The model under review builds one solid part; all positions refer to its coordinate system, in mm. A direction names the side the tool comes from. Round coordinates to 2 decimals unless told otherwise and drop trailing zeros. Order: outer loops, then holes, each group sorted by start corner. A loop starts at its lowest first (then second) coordinate and runs counter-clockwise, first axis right, second up.
from build123d import *

# Parameters (mm, degrees)
ROTATION1_ANGLE                                      = 180
FORMSENKUNG_F_R_M3_SENKSCHRAUBE_MIT_INNE_D           = 1.6
FORMSENKUNG_F_R_M3_SENKSCHRAUBE_MIT_INNE_DEPTH       = 12
FORMSENKUNG_F_R_M3_SENKSCHRAUBE_MIT_INNE_CSINK_D     = 3.9
FORMSENKUNG_F_R_M3_SENKSCHRAUBE_MIT_INNE_CSINK_ANGLE = 90
FORMSENKUNG_F_R_M3_SENKSCHRAUBE_MIT_INNE_TIP         = 0.480688495
SKIZZE12_R                                           = 1
SCHNITT_LINEAR_AUSTRAGEN1_DEPTH                      = 10.5
SKIZZE9_R                                            = 3
SCHNITT_LINEAR_AUSTRAGEN2_DEPTH                      = 19
SKIZZE9_5_R                                          = 3.5
SCHNITT_LINEAR_AUSTRAGEN3_DEPTH                      = 16.5
SCHNITT_LINEAR_AUSTRAGEN5_DEPTH                      = 4
STIRNSENKUNG_F_R_M3_D_NNKOPF_ZYLINDERSCH_D           = 3.2
STIRNSENKUNG_F_R_M3_D_NNKOPF_ZYLINDERSCH_CBORE_D     = 5.6
STIRNSENKUNG_F_R_M3_D_NNKOPF_ZYLINDERSCH_CBORE_DEPTH = 2.1


with BuildPart() as part:
    # Skizze4 → Rotation1 (revolve, symmetric)
    with BuildSketch(Plane.XY) as rotation1_sk:
        Polygon((3.5, 20), (-4, 20), (-4, 13), (5.5, 13), (5.5, 22), (3.5, 22), align=None)
    revolve(axis=Axis((0, 0, 0), (-1, 0, 0)), revolution_arc=ROTATION1_ANGLE / 2)
    revolve(rotation1_sk.sketch, axis=Axis((0, 0, 0), (1, 0, 0)), revolution_arc=ROTATION1_ANGLE / 2)

    # Formsenkung f_r M3 Senkschraube mit Inne
    with Locations(Plane(origin=(5.5, 0, 0), x_dir=(0, 0, -1), z_dir=(1, 0, 0))):
        with Locations((6.696960066, 16.167891819), (-16.167891819, 6.696960066), (-6.696960066, 16.167891819), (16.167891819, 6.696960066)):
            CounterSinkHole(FORMSENKUNG_F_R_M3_SENKSCHRAUBE_MIT_INNE_D / 2, FORMSENKUNG_F_R_M3_SENKSCHRAUBE_MIT_INNE_CSINK_D / 2, depth=FORMSENKUNG_F_R_M3_SENKSCHRAUBE_MIT_INNE_DEPTH, counter_sink_angle=FORMSENKUNG_F_R_M3_SENKSCHRAUBE_MIT_INNE_CSINK_ANGLE)
            with Locations((0, 0, -(FORMSENKUNG_F_R_M3_SENKSCHRAUBE_MIT_INNE_DEPTH + FORMSENKUNG_F_R_M3_SENKSCHRAUBE_MIT_INNE_TIP / 2))):  # 118° drill point
                Cone(0, FORMSENKUNG_F_R_M3_SENKSCHRAUBE_MIT_INNE_D / 2, FORMSENKUNG_F_R_M3_SENKSCHRAUBE_MIT_INNE_TIP, mode=Mode.SUBTRACT)

    # Skizze12 → Schnitt-Linear austragen1 (cut, through all)
    with BuildSketch(Plane(origin=(5.5, 0, 0), x_dir=(0, 0, -1), z_dir=(1, 0, 0))):
        with Locations((-6.696960066, 16.167891819)):
            Circle(SKIZZE12_R)
        with Locations((6.696960066, 16.167891819)):
            Circle(SKIZZE12_R)
        with Locations((16.167891819, 6.696960066)):
            Circle(SKIZZE12_R)
        with Locations((-16.167891819, 6.696960066)):
            Circle(SKIZZE12_R)
    extrude(amount=-SCHNITT_LINEAR_AUSTRAGEN1_DEPTH, mode=Mode.SUBTRACT)

    # Skizze9 → Schnitt-Linear austragen2 (cut, symmetric)
    with BuildSketch(Plane(origin=(0, 0, 0), x_dir=(1, 0, 0), z_dir=(0, 1, 0))):
        Circle(SKIZZE9_R)
    extrude(amount=SCHNITT_LINEAR_AUSTRAGEN2_DEPTH, both=True, mode=Mode.SUBTRACT)

    # Skizze9_5 → Schnitt-Linear austragen3 (cut, symmetric)
    with BuildSketch(Plane(origin=(0, 0, 0), x_dir=(1, 0, 0), z_dir=(0, 1, 0))):
        Circle(SKIZZE9_5_R)
    extrude(amount=SCHNITT_LINEAR_AUSTRAGEN3_DEPTH, both=True, mode=Mode.SUBTRACT)

    # Skizze15 → Schnitt-Linear austragen5 (cut)
    with BuildSketch(Plane(origin=(5.5, 0, 0), x_dir=(0, 0, -1), z_dir=(1, 0, 0))):
        Polygon((-14.883419246, 2.8), (-18.116580754, 2.8), (-19.733161507, 0), (-18.116580754, -2.8), (-14.883419246, -2.8), (-13.266838493, 0), align=None)
        Polygon((13.266838493, 0), (14.883419246, 2.8), (18.116580754, 2.8), (19.733161507, 0), (18.116580754, -2.8), (14.883419246, -2.8), align=None)
    extrude(amount=-SCHNITT_LINEAR_AUSTRAGEN5_DEPTH, mode=Mode.SUBTRACT)

    # Stirnsenkung f_r M3 D_nnkopf-Zylindersch (through all)
    with Locations(Plane.ZY.offset(4)):
        with Locations((16.5, 0), (-16.5, 0)):
            CounterBoreHole(STIRNSENKUNG_F_R_M3_D_NNKOPF_ZYLINDERSCH_D / 2, STIRNSENKUNG_F_R_M3_D_NNKOPF_ZYLINDERSCH_CBORE_D / 2, STIRNSENKUNG_F_R_M3_D_NNKOPF_ZYLINDERSCH_CBORE_DEPTH)


solid = part.part
(1) We need section C-C (y = 20.75). Give the boundary of the cut face in (x, z), and give its area (3 significant figures).
(2) We need section A-A (z = 0). Give the boundary of the cut face in (x, y), and give its area (3 significant figures).
(3) We need section D-D (z = 12.5). Give the boundary of the cut face in (x, y).
(4) Clearance check with flat-ended pins moving along their axes: P1, Ø6, axis at y = 3.5, z = -6.5, coming from the -X side; P2, Ø2.5, axis at y = 16.17, z = 6.7, coming from the +X side; P3, Ø4, axis at x = 0, z = 0, coming from the +Y side; P4, Ø5, axis at x = 3.5, z = 3, coming from the -Y side. State where each tip first meets the part, or that it passes through.
(5) To check wall thickness, follow L1, parallel to Z at x = 0, y = 15.4; L2, parallel to Z at x = 2.5, y = 7 (3 decimals); L3, parallel to X at y = 18.35, z = 0. State the ranges of each line that lie inside material, in increasing order.
(6) We need section B-B (x = 0). Give the boundary of the cut face in (y, z).
(7) The part is to be moulded in two halves that separate along Z. For faces 1 (the flat face through (0, 0, 14)), 2 (the cylindrical face through (4, 22, 0)), 3 (the cylindrical face through (3.34, 14.54, -1.05)), 4 (the flat face through (1.5, 2, -17)), say which applies: pulls with the +Z half, pulls with the -Z half, needs draft (parallel to the pull), parting line crosses it, or undercut.
(8) Tool access review of faces 5 (the cylindrical face through (-3, 2.8, 16.6)), 6 (the flat face through (3.5, 20, -3)), 7 (the flat face through (3.528, 1.42, 18.914)), 8 (the cylindrical face through (0.33, 6.74, -15.17)), 9 (the flat face through (0, 19, 0)): name each direction out of +Z, -Z, +X, -X, +Y, -Y from which nothing blocks a thin tool from reaching the whole face with its end or side.
Verdict:
1. outline: (3.5, -7.31) - (5.5, -7.31) - (5.5, 7.31) - (3.5, 7.31) - close
1. area: 29.2 mm2
2. outline: (-4, 13) - (-3.5, 13) - (-3.5, 16.5) - (-3, 16.5) - (-3, 19) - (3, 19) - (3, 16.5) - (3.5, 16.5) - (3.5, 13) - (5.5, 13) - (5.5, 22) - (3.5, 22) - (3.5, 20) - (-4, 20) - close
2. area: 31.0 mm2
3. outline: (-4, 3.57) - (5.5, 3.57) - (5.5, 18.1) - (3.5, 18.1) - (3.5, 15.61) - (-4, 15.61) - close
4. P1: passes through
4. P2: stops at x = 4.8
4. P3: stops at y = 20
4. P4: stops at y = 11.78
5. L1: z = -12.76 to -7.34, -6.06 to -3.5, 3.5 to 6.06, 7.34 to 12.76
5. L2: z = -18.735 to -17.121, -15.215 to -10.954, 10.954 to 15.215, 17.121 to 18.735
5. L3: x = -4 to -3, 3 to 5.5
6. outline: (0, -20) arc R20 ccw to (0, 20) - (0, 18.1) arc R1.6 cw to (0, 14.9) - (0, 13) arc R13 cw to (12.52, 3.5) - (16.5, 3.5) - (16.5, 3) - (19, 3) - (19, -3) - (16.5, -3) - (16.5, -3.5) - (12.52, -3.5) arc R13 cw to (0, -13) - (0, -14.9) arc R1.6 cw to (0, -18.1) - close; hole circle Ø2 at (6.7, -16.17); hole circle Ø2 at (6.7, 16.17); hole circle Ø2 at (16.17, -6.7); hole circle Ø2 at (16.17, 6.7)
7. face 1: needs draft
7. face 2: parting line crosses it
7. face 3: undercut
7. face 4: undercut
8. face 5: -X, -Y
8. face 6: -X, +Y
8. face 7: +X, -Y
8. face 8: +X, -X
8. face 9: -Y
